Design review of the part shown in the three views and the two pictorial views. Dimensions are in mm from the part's minimum x, y and z. Round coordinates to 2 decimals unless told otherwise and drop trailing zeros. Order: outer loops, then holes, each group sorted by start corner. A loop starts at its lowest first (then second) coordinate and runs counter-clockwise, first axis right, second up. Notation, with made-up numbers: (27.25, 6.5) - (53.25, 6.5) arc R19 cw to (53.25, 25.5) - close; hole circle Ø11 at (35.5, -20.75). An arc over 180 degrees is marked (long way). Use CSV: the item, a comma, the result in double quotes.
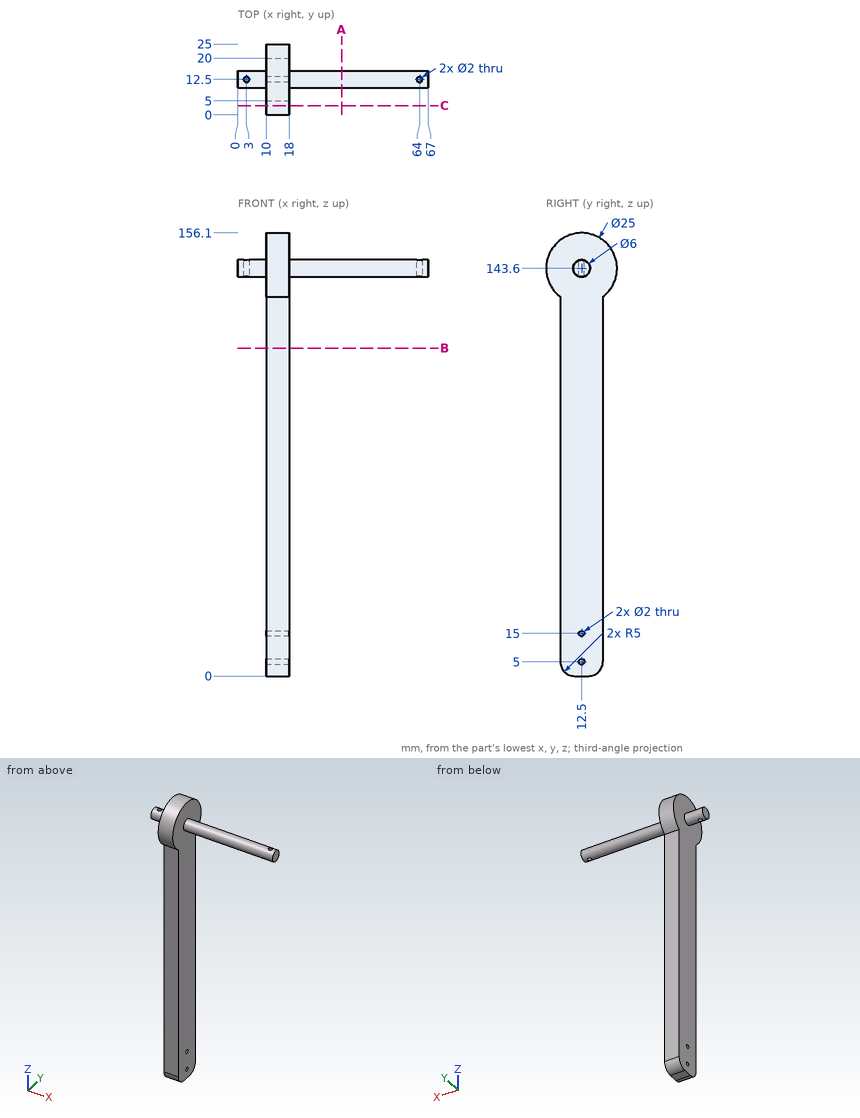
1) We need section A-A (x = 36.5). Give the boundary of the cut face in (y, z).
Data:
outline,"circle Ø6 at (12.5, 143.6)"
2) Insertion check: pin 1 Ø2.5 at (y, z) = (12.5, 15) entering from +X; pin 2 Ø4 at (x, z) = (18, 40) entering from +Y; pin 3 Ø1.8 at (y, z) = (12.5, 5) entering from -X; pin 4 Ø2.5 at (x, y) = (3, 12.5) entering from -Z. Each pin has a flat end and moves straight along its axis. Give the tip position at first contact, or say it passes through.
Data:
pin 1,"stops at x = 18"
pin 2,"stops at y = 20"
pin 3,"passes through"
pin 4,"stops at z = 140.6"
3) We need section B-B (z = 115.5). Give the boundary of the cut face in (x, y), then the cut area to 3 significant figures.
Data:
outline,"(10, 5) - (18, 5) - (18, 20) - (10, 20) - close"
area,"120 mm2"
4) To check wall thickness, follow L1, parallel to X at y = 12.5, z = 145; L2, parallel to Y at x = 13, z = 15; L3, parallel to Y at x = 3, z = 144. State the ranges of each line that lie inside material, in increasing order. Write a range as from..to.
Data:
L1,"x = 0..2, 4..63, 65..67"
L2,"y = 5..11.5, 13.5..20"
L3,"y = 9.53..11.5, 13.5..15.47"
5) We need section C-C (y = 3.25). Give the boundary of the cut face in (x, z).
Data:
outline,"(10, 135.19) - (18, 135.19) - (18, 152.01) - (10, 152.01) - close"
